from build123d import *

# Parameters (mm, degrees)
ESQUISSE1_W         = 590.5
ESQUISSE1_H         = 280
BOSS_EXTRUDE1_DEPTH = 18
CUT_EXTRUDE1_DEPTH  = 654.769263579
ESQUISSE3_R         = 5
CUT_EXTRUDE2_DEPTH  = 654.769263579
CONG_1_R            = 7


with BuildPart() as part:
    # Esquisse1 → Boss-Extrude1 (new body)
    with BuildSketch(Plane.XY):
        with Locations((295.25, 140)):
            Rectangle(ESQUISSE1_W, ESQUISSE1_H)
    extrude(amount=BOSS_EXTRUDE1_DEPTH)

    # Esquisse2 → Cut-Extrude1 (cut, through all)
    with BuildSketch(Plane.XY.offset(18)):
        with BuildLine():
            Line((69.477649355, 140), (78.147350645, 140))
            ThreePointArc((78.147350645, 140), (78.480108702, 140.056987765), (78.774940482, 140.221455848))
            ThreePointArc((78.774940482, 140.221455848), (82.906692971, 140.005791686), (83.14421642, 135.875238181))
            ThreePointArc((83.14421642, 135.875238181), (82.981710298, 135.580689894), (82.926074516, 135.248919502))
            Line((82.926074516, 135.248919502), (83.3125, 0))
            Line((83.3125, 0), (64.3125, 0))
            Line((64.3125, 0), (64.698925484, 135.248919502))
            ThreePointArc((64.698925484, 135.248919502), (64.643289702, 135.580689894), (64.48078358, 135.875238181))
            ThreePointArc((64.48078358, 135.875238181), (64.718307029, 140.005791686), (68.850059518, 140.221455848))
            ThreePointArc((68.850059518, 140.221455848), (69.144891298, 140.056987765), (69.477649355, 140))
        make_face()
    extrude(amount=-CUT_EXTRUDE1_DEPTH, mode=Mode.SUBTRACT)

    # Esquisse3 → Cut-Extrude2 (cut, through all)
    with BuildSketch(Plane.XY.offset(18)):
        with Locations((422.0625, 233.333333333)):
            Circle(ESQUISSE3_R)
    extrude(amount=-CUT_EXTRUDE2_DEPTH, mode=Mode.SUBTRACT)

    # Cong_1
    cong_1_edges = [part.edges().sort_by_distance(p)[0] for p in [
        (83.3125, 0, 9),
        (64.3125, 0, 9),
        (0, 280, 9),
        (0, 0, 9),
    ]]
    fillet(cong_1_edges, radius=CONG_1_R)

    # Sym_trie1: part across plane


with BuildPart() as part_1:
    add(part.part)
    add(part.part.mirror(Plane(origin=(590.5, 0, 18), x_dir=(0, 0, 1), z_dir=(-1, 0, 0))))


solid = part_1.part
Model file for the job. Use its own axes, mm. Give positions to 0.01 mm unless a question says otherwise; leave off trailing zeros. Loops run counter-clockwise (first coordinate to the right, second up) from the corner with the lowest first, then second, coordinate; pieces in that order, holes last.
1) Wall check: line 1 (X direction, y = 89.5, z = 15); line 2 (X direction, y = 72, z = 15.75); line 3 (Y direction, x = 70.5, z = 16.5). Give the ranges that are in metal, low to high.
2) Saw through at C-C (y = 37.5). Write the cut outline in (x, z).
3) Saw through at A-A (y = 101). Write the cut outline in (x, z), plus the area to 3 significant figures.
4) Saw through at B-B (z = 9.75). Count the separate pieces of the cut face and the enclosed holes in it, plus the area to 3 significant figures.
5) Flat gauge pins, fed straight in: pin 1 Ø4.5 at (x, z) = (74.5, 10.5) entering from -Y; pin 2 Ø6 at (x, y) = (422.06, 233.33) entering from -Z. Where does each tip first touch, or does it go through?
Answer block:
1. line 1: x = 0 to 64.57, 83.06 to 1097.94, 1116.43 to 1181
1. line 2: x = 0 to 64.52, 83.11 to 1097.89, 1116.48 to 1181
1. line 3: y = 140 to 280
2. outline: (0, 0) - (64.42, 0) - (64.42, 18) - (0, 18) - close; (83.21, 0) - (1097.79, 0) - (1097.79, 18) - (83.21, 18) - close; (1116.58, 0) - (1181, 0) - (1181, 18) - (1116.58, 18) - close
3. outline: (0, 0) - (64.6, 0) - (64.6, 18) - (0, 18) - close; (83.02, 0) - (1097.98, 0) - (1097.98, 18) - (83.02, 18) - close; (1116.4, 0) - (1181, 0) - (1181, 18) - (1116.4, 18) - close
3. area: 20,600 mm2
4. separate pieces: 1
4. enclosed holes: 2
4. area: 325,000 mm2
5. pin 1: stops at y = 140
5. pin 2: passes through
